Input: part model. Units: mm. Frame: model coordinates. Round coordinates to 2 decimals unless told otherwise and drop trailing zeros. Order: outer loops, then holes, each group sorted by start corner. A loop starts at its lowest first (then second) coordinate and runs counter-clockwise, first axis right, second up. Notation, with made-up numbers: (23, 8) -> (47, 8) arc R38 ccw to (47, 46) -> close; hole circle Ø3 at (64.5, 35.25). An arc over 180 degrees is marked (long way). Answer as CSV lines item,"result". Start each with the question number.
1) Section query C-C, the plane z = 0.95. State how many separate pieces and enclosed holes the cut face has, and give its area (3 significant figures).
2) Line query: L1, parallel to Y at x = 79, z = 1.1; L2, parallel to Y at x = -91.5, z = 2.05; L3, parallel to X at y = 83, z = 2.75. Output: solid intervals per line, ascending.
3) Section query A-A, the plane x = 68. Output: boundary loops of the cut face in (y, z), and give its area (3 significant figures).
4) Section query B-B, the plane x = -14. Output: boundary loops of the cut face in (y, z), and give its area (3 significant figures).
```python
from build123d import *

# Parameters (mm, degrees)
SKETCH1_W           = 300
SKETCH1_H           = 200
BOSS_EXTRUDE1_DEPTH = 3
CUT_EXTRUDE1_DEPTH  = 3
CUT_EXTRUDE2_DEPTH  = 10
CUT_EXTRUDE3_DEPTH  = 10
CUT_EXTRUDE4_DEPTH  = 10
CUT_EXTRUDE5_DEPTH  = 10
CUT_EXTRUDE6_DEPTH  = 10
CUT_EXTRUDE7_DEPTH  = 10
CUT_EXTRUDE8_DEPTH  = 10
SKETCH10_W          = 300
SKETCH10_H          = 3
BOSS_EXTRUDE2_DEPTH = 40


with BuildPart() as part:
    # Sketch1 → Boss-Extrude1 (new body)
    with BuildSketch(Plane.XY):
        Rectangle(SKETCH1_W, SKETCH1_H)
    extrude(amount=BOSS_EXTRUDE1_DEPTH)

    # Sketch2 → Cut-Extrude1 (cut)
    with BuildSketch(Plane(origin=(0, 0, 0), x_dir=(-1, 0, 0), z_dir=(0, 0, -1))):
        with BuildLine():
            Line((-100, -23), (100, -23))
            ThreePointArc((100, -23), (102, -25), (100, -27))
            Line((100, -27), (-100, -27))
            ThreePointArc((-100, -27), (-102, -25), (-100, -23))
        make_face()
        with BuildLine():
            Line((-100, 7), (100, 7))
            ThreePointArc((100, 7), (102, 5), (100, 3))
            Line((100, 3), (-100, 3))
            ThreePointArc((-100, 3), (-102, 5), (-100, 7))
        make_face()
        with BuildLine():
            Line((-50, 26), (100, 26))
            ThreePointArc((100, 26), (102, 24), (100, 22))
            Line((100, 22), (-50, 22))
            ThreePointArc((-50, 22), (-52, 24), (-50, 26))
        make_face()
        with BuildLine():
            Line((-50, 90), (100, 90))
            ThreePointArc((100, 90), (102, 88), (100, 86))
            Line((100, 86), (-50, 86))
            ThreePointArc((-50, 86), (-52, 88), (-50, 90))
        make_face()
    extrude(amount=-CUT_EXTRUDE1_DEPTH, mode=Mode.SUBTRACT)

    # Sketch3 → Cut-Extrude2 (cut)
    with BuildSketch(Plane(origin=(0, 0, 0), x_dir=(-1, 0, 0), z_dir=(0, 0, -1))):
        with BuildLine():
            Line((143.044786866, 93), (143.044786866, 83))
            ThreePointArc((143.044786866, 83), (141.044786866, 81), (139.044786866, 83))
            Line((139.044786866, 83), (139.044786866, 93))
            ThreePointArc((139.044786866, 93), (141.044786866, 95), (143.044786866, 93))
        make_face()
    extrude(amount=-CUT_EXTRUDE2_DEPTH, mode=Mode.SUBTRACT)

    # Sketch4 → Cut-Extrude3 (cut)
    with BuildSketch(Plane(origin=(0, 0, 0), x_dir=(-1, 0, 0), z_dir=(0, 0, -1))):
        with BuildLine():
            Line((144.5, -83), (144.5, -93))
            ThreePointArc((144.5, -93), (142.5, -95), (140.5, -93))
            Line((140.5, -93), (140.5, -83))
            ThreePointArc((140.5, -83), (142.5, -81), (144.5, -83))
        make_face()
    extrude(amount=-CUT_EXTRUDE3_DEPTH, mode=Mode.SUBTRACT)

    # Sketch5 → Cut-Extrude4 (cut)
    with BuildSketch(Plane(origin=(0, 0, 0), x_dir=(-1, 0, 0), z_dir=(0, 0, -1))):
        with BuildLine():
            Line((-140.5, 93), (-140.5, 83))
            ThreePointArc((-140.5, 83), (-142.5, 81), (-144.5, 83))
            Line((-144.5, 83), (-144.5, 93))
            ThreePointArc((-144.5, 93), (-142.5, 95), (-140.5, 93))
        make_face()
    extrude(amount=-CUT_EXTRUDE4_DEPTH, mode=Mode.SUBTRACT)

    # Sketch6 → Cut-Extrude5 (cut)
    with BuildSketch(Plane(origin=(0, 0, 0), x_dir=(-1, 0, 0), z_dir=(0, 0, -1))):
        with BuildLine():
            Line((-140.5, -83), (-140.5, -93))
            ThreePointArc((-140.5, -93), (-142.5, -95), (-144.5, -93))
            Line((-144.5, -93), (-144.5, -83))
            ThreePointArc((-144.5, -83), (-142.5, -81), (-140.5, -83))
        make_face()
    extrude(amount=-CUT_EXTRUDE5_DEPTH, mode=Mode.SUBTRACT)

    # Sketch7 → Cut-Extrude6 (cut)
    with BuildSketch(Plane(origin=(0, 0, 0), x_dir=(-1, 0, 0), z_dir=(0, 0, -1))):
        with BuildLine():
            Line((2, -83), (2, -93))
            ThreePointArc((2, -93), (0, -95), (-2, -93))
            Line((-2, -93), (-2, -83))
            ThreePointArc((-2, -83), (0, -81), (2, -83))
        make_face()
    extrude(amount=-CUT_EXTRUDE6_DEPTH, mode=Mode.SUBTRACT)

    # Sketch8 → Cut-Extrude7 (cut)
    with BuildSketch(Plane(origin=(0, 0, 0), x_dir=(-1, 0, 0), z_dir=(0, 0, -1))):
        with BuildLine():
            Line((-143, 65), (-133, 65))
            ThreePointArc((-133, 65), (-131, 63), (-133, 61))
            Line((-133, 61), (-143, 61))
            ThreePointArc((-143, 61), (-145, 63), (-143, 65))
        make_face()
        with BuildLine():
            Line((-143, -61), (-133, -61))
            ThreePointArc((-133, -61), (-131, -63), (-133, -65))
            Line((-133, -65), (-143, -65))
            ThreePointArc((-143, -65), (-145, -63), (-143, -61))
        make_face()
        with BuildLine():
            Line((-143, 2), (-133, 2))
            ThreePointArc((-133, 2), (-131, 0), (-133, -2))
            Line((-133, -2), (-143, -2))
            ThreePointArc((-143, -2), (-145, 0), (-143, 2))
        make_face()
    extrude(amount=-CUT_EXTRUDE7_DEPTH, mode=Mode.SUBTRACT)

    # Sketch9 → Cut-Extrude8 (cut)
    with BuildSketch(Plane(origin=(0, 0, 0), x_dir=(-1, 0, 0), z_dir=(0, 0, -1))):
        with BuildLine():
            Line((133, 65), (143, 65))
            ThreePointArc((143, 65), (145, 63), (143, 61))
            Line((143, 61), (133, 61))
            ThreePointArc((133, 61), (131, 63), (133, 65))
        make_face()
        with BuildLine():
            Line((133, 2), (143, 2))
            ThreePointArc((143, 2), (145, 0), (143, -2))
            Line((143, -2), (133, -2))
            ThreePointArc((133, -2), (131, 0), (133, 2))
        make_face()
        with BuildLine():
            Line((133, -61), (143, -61))
            ThreePointArc((143, -61), (145, -63), (143, -65))
            Line((143, -65), (133, -65))
            ThreePointArc((133, -65), (131, -63), (133, -61))
        make_face()
    extrude(amount=-CUT_EXTRUDE8_DEPTH, mode=Mode.SUBTRACT)

    # Sketch10 → Boss-Extrude2 (add)
    with BuildSketch(Plane(origin=(0, 100, 0), x_dir=(1, 0, 0), z_dir=(0, 1, 0))):
        with Locations((0, -1.5)):
            Rectangle(SKETCH10_W, SKETCH10_H)
    extrude(amount=BOSS_EXTRUDE2_DEPTH)


solid = part.part
```
Findings:
1,separate pieces,"1"
1,enclosed holes,"15"
1,area,"68,600 mm^2"
2,L1,"y = -100 to -27, -23 to 3, 7 to 140"
2,L2,"y = -100 to -27, -23 to 3, 7 to 22, 26 to 86, 90 to 140"
2,L3,"x = -150 to -143.04, -139.04 to 140.5, 144.5 to 150"
3,outline,"(-100, 0) -> (-27, 0) -> (-27, 3) -> (-100, 3) -> close; (-23, 0) -> (3, 0) -> (3, 3) -> (-23, 3) -> close; (7, 0) -> (140, 0) -> (140, 3) -> (7, 3) -> close"
3,area,"696 mm^2"
4,outline,"(-100, 0) -> (-27, 0) -> (-27, 3) -> (-100, 3) -> close; (-23, 0) -> (3, 0) -> (3, 3) -> (-23, 3) -> close; (7, 0) -> (22, 0) -> (22, 3) -> (7, 3) -> close; (26, 0) -> (86, 0) -> (86, 3) -> (26, 3) -> close; (90, 0) -> (140, 0) -> (140, 3) -> (90, 3) -> close"
4,area,"672 mm^2"
